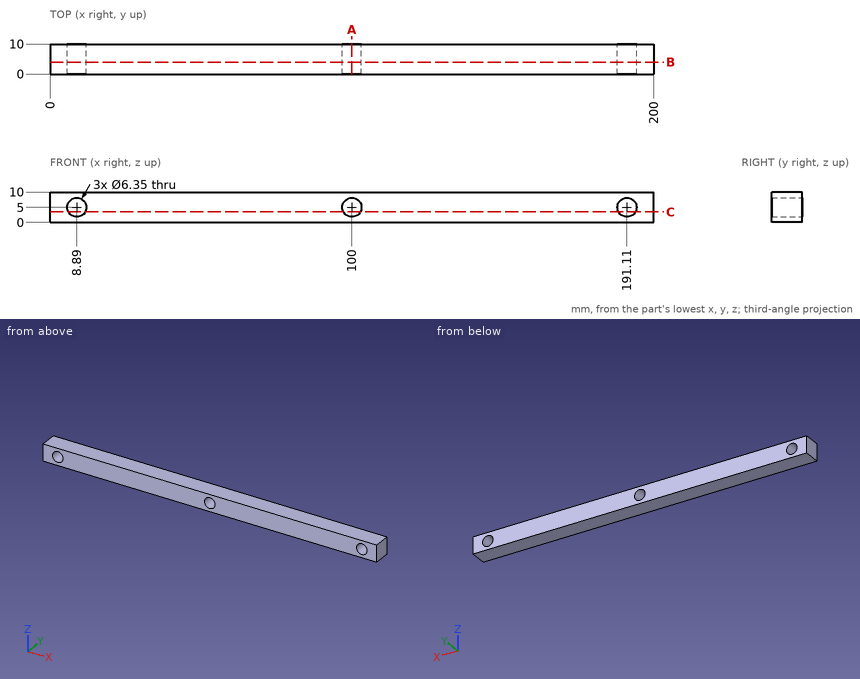
Print and shaded views of the part. All mm, measured from the part's lowest x, y and z. Round coordinates to 2 decimals unless told otherwise and drop trailing zeros. Write each loop counter-clockwise with the first axis right and the second up, starting at its lowest first coordinate (ties: lowest second). Pieces come first, ordered by that corner, then holes. Notation, with made-up numbers: (-36, 41) -> (-23, 41) arc R16 ccw to (-23, 70) -> close; hole circle Ø1 at (16, 38.25). An arc over 180 degrees is marked (long way). Return JSON: item names as keys, results as strings. Group by question number.
Q1. Saw through at C-C on z = 3.5. Write the cut outline in (x, y), plus the area to 3 significant figures.
Q2. Saw through at B-B on y = 4. Write the cut outline in (x, z) (3 decimals), plus the area to 3 significant figures.
Q3. Pin check, flat tip, straight feed: pin 1 (4 mm diameter, centred on x = 104.5, y = 3.5, fed in from -Z). Stop position of the tip, or through.
Q4. Probe L1, parallel to X at y = 4.5, z = 5.5; L2, parallel to X at y = 9.5, z = 5.25; L3, parallel to Z at x = 191.11, y = 3.25 (3 decimals). List the from-to ranges inside material, lowest first. Write a range as [from, to].
Q5. Saw through at A-A on x = 100. Write the cut outline in (y, z) (3 decimals).
Answer:
{
 "1": {"outline": "(0, 0) -> (6.09, 0) -> (6.09, 10) -> (0, 10) -> close; (11.69, 0) -> (97.2, 0) -> (97.2, 10) -> (11.69, 10) -> close; (102.8, 0) -> (188.31, 0) -> (188.31, 10) -> (102.8, 10) -> close; (193.91, 0) -> (200, 0) -> (200, 10) -> (193.91, 10) -> close", "area": "1,830 mm2"},
 "2": {"outline": "(0, 0) -> (200, 0) -> (200, 10) -> (0, 10) -> close; hole circle Ø6.35 at (8.89, 5); hole circle Ø6.35 at (100, 5); hole circle Ø6.35 at (191.11, 5)", "area": "1,900 mm2"},
 "3": {"pin 1": "z = 0"},
 "4": {"L1": "[0, 5.75], [12.03, 96.86], [103.14, 187.97], [194.25, 200]", "L2": "[0, 5.72], [12.06, 96.83], [103.17, 187.94], [194.28, 200]", "L3": "[0, 1.825], [8.175, 10]"},
 "5": {"outline": "(0, 0) -> (10, 0) -> (10, 1.825) -> (0, 1.825) -> close; (0, 8.175) -> (10, 8.175) -> (10, 10) -> (0, 10) -> close"}
}
